Read the model definition and answer for the solid it produces. Units are mm, in the model's axes. Face numbers are marked on the shaded views. A direction names the side the tool comes from. Give positions to 0.01 mm unless a question says otherwise; leave off trailing zeros. Order: outer loops, then holes, each group sorted by start corner. A loop starts at its lowest first (then second) coordinate and runs counter-clockwise, first axis right, second up.
Item 1: Given pin 1 Ø1.5 at (y, z) = (32, 19.5) entering from +X; pin 2 Ø5 at (x, y) = (56, 18) entering from -Z; pin 3 Ø10 at (x, y) = (57.5, 44) entering from +Z; pin 4 Ø6 at (x, z) = (21.5, 40.5) entering from -Y, each flat-ended and moving along its own axis, determine where each tip first touches the part or whether it passes through.
Item 2: Find the intervals of material crossed by line 1 along X through (y, z) = (32, 18); line 2 along Z through (x, y) = (29, 38); line 3 along Y through (x, z) = (3.5, 25.5), in increasing order.
Item 3: A cutting plane is placed at C-C (z = 18). Write down the section's boundary in (x, y).
Item 4: Which of the six approach directions +Z, -Z, +X, -X, +Y, -Y give full straight-line access (tool end or side, diameter ignored) to the marked faces 1 and 2?
Item 5: A cutting plane is placed at B-B (y = 11.5). Write down the section's boundary in (x, z), plus the area to 3 significant figures.
Item 6: A cutting plane is placed at A-A (x = 13). Write down the section's boundary in (y, z).
Item 7: A cutting plane is placed at D-D (x = 41.5). Write down the section's boundary in (y, z).
from build123d import *

# Parameters (mm, degrees)
F2_DEPTH = 50.8
F3_DEPTH = 25.4


with BuildPart() as f2:
    # F0 (on Front) → F2 (new body)
    with BuildSketch(Plane.XZ):
        Polygon((0, 50.8), (0, 0), (76.2, 0), (76.2, 12.7), (25.4, 12.7), (25.4, 50.8), align=None)
    extrude(amount=-F2_DEPTH)

    # F1 (on Right) → F3 (cut)
    with BuildSketch(Plane.YZ):
        with BuildLine():
            Line((50.8, 50.8), (25.4, 50.8))
            ThreePointArc((25.4, 50.8), (43.360512, 43.360512), (50.8, 25.4))
            Line((50.8, 25.4), (50.8, 50.8))
        make_face()
        with BuildLine():
            ThreePointArc((0, 25.4), (7.439488, 43.360512), (25.4, 50.8))
            Line((25.4, 50.8), (0, 50.8))
            Line((0, 50.8), (0, 25.4))
        make_face()
    extrude(amount=F3_DEPTH, mode=Mode.SUBTRACT)


solid = f2.part
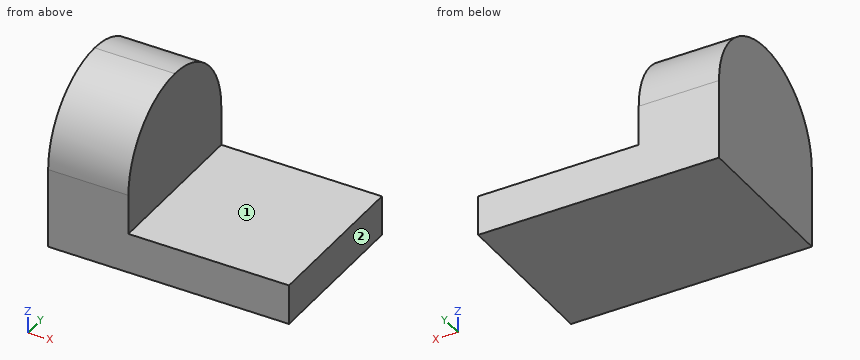
Response values:
1. pin 1: stops at x = 25.4
1. pin 2: stops at z = 0
1. pin 3: stops at z = 12.7
1. pin 4: stops at y = 3.07
2. line 1: x = 0 to 25.4
2. line 2: z = 0 to 12.7
2. line 3: y = 0 to 50.8
3. outline: (0, 0) - (25.4, 0) - (25.4, 50.8) - (0, 50.8) - close
4. face 1: +Z, +X, +Y, -Y
4. face 2: +Z, -Z, +X, +Y, -Y
5. outline: (0, 0) - (76.2, 0) - (76.2, 12.7) - (25.4, 12.7) - (25.4, 46.66) - (0, 46.66) - close
5. area: 1,830 mm2
6. outline: (0, 0) - (50.8, 0) - (50.8, 25.4) arc R25.4 ccw to (25.4, 50.8) arc R25.4 ccw to (0, 25.4) - close
7. outline: (0, 0) - (50.8, 0) - (50.8, 12.7) - (0, 12.7) - close
